Source: CAD feature listing. Evaluate the final solid. Frame: model axes, mm. A direction names the side the tool comes from. Give positions to 0.01 mm unless a question says otherwise; leave off trailing zeros. Order: outer loops, then holes, each group sorted by start corner. A loop starts at its lowest first (then second) coordinate and runs counter-clockwise, first axis right, second up. Notation, with made-up numbers: (87.5, 27) - (121.5, 27) arc R29 cw to (121.5, 63) - close; hole circle Ø4 at (76.5, 73). An arc over 180 degrees is marked (long way). Answer as CSV lines item,"result".
```python
from build123d import *

# Parameters (mm, degrees)
SCHIZZO2_R                    = 10.5
ESTRUSIONE_ESTRUSIONE1_DEPTH  = 22
TAGLIO_ESTRUSIONE1_DEPTH      = 17
SMUSSO1_SIZE                  = 2
TAGLIO_ESTRUSIONE2_DEPTH      = 27.54241888
TAGLIO_ESTRUSIONE2_DEPTH_BACK = 27.54241888
SCHIZZO4_R                    = 2
TAGLIO_ESTRUSIONE3_DEPTH      = 27.542418959
TAGLIO_ESTRUSIONE3_DEPTH_BACK = 19
SCHIZZO5_R                    = 0.9


with BuildPart() as part:
    # Schizzo2 → Estrusione-Estrusione1 (new body)
    with BuildSketch(Plane(origin=(0, 0, 0), x_dir=(1, 0, 0), z_dir=(0, 1, 0))):
        with Locations(Location((0, 0, 0), (0, 0, 270))):
            Circle(SCHIZZO2_R)
    extrude(amount=ESTRUSIONE_ESTRUSIONE1_DEPTH)

    # Schizzo3 → Taglio-Estrusione1 (cut)
    with BuildSketch(Plane.XZ):
        with BuildLine():
            Line((-2.860934268, 7.5), (2.860934268, 7.5))
            ThreePointArc((2.860934268, 7.5), (4.373482153, 6.873482153), (5, 5.360934268))
            Line((5, 5.360934268), (5, -5.360934268))
            ThreePointArc((5, -5.360934268), (4.373482153, -6.873482153), (2.860934268, -7.5))
            Line((2.860934268, -7.5), (-2.860934268, -7.5))
            ThreePointArc((-2.860934268, -7.5), (-4.373482153, -6.873482153), (-5, -5.360934268))
            Line((-5, -5.360934268), (-5, 5.360934268))
            ThreePointArc((-5, 5.360934268), (-4.373482153, 6.873482153), (-2.860934268, 7.5))
        make_face()
    extrude(amount=-TAGLIO_ESTRUSIONE1_DEPTH, mode=Mode.SUBTRACT)

    # Smusso1
    smusso1_edges = [part.edges().sort_by_distance(p)[0] for p in [
        (0, 22, -10.5),
    ]]
    chamfer(smusso1_edges, length=SMUSSO1_SIZE)

    # Schizzo4 → Taglio-Estrusione2 (cut, two sides: drawn at the far end of the back side and taken through both)
    with BuildSketch(Plane(origin=(0, 0, 0), x_dir=(0, 0, -1), z_dir=(1, 0, 0)).offset(-TAGLIO_ESTRUSIONE2_DEPTH_BACK)):
        with Locations(Location((0, 10, 0), (0, 0, 270))):
            Circle(SCHIZZO4_R)
    extrude(amount=TAGLIO_ESTRUSIONE2_DEPTH + TAGLIO_ESTRUSIONE2_DEPTH_BACK, mode=Mode.SUBTRACT)

    # Schizzo5 → Taglio-Estrusione3 (cut, two sides: drawn at the far end of the back side and taken through both)
    with BuildSketch(Plane.XZ.offset(-TAGLIO_ESTRUSIONE3_DEPTH_BACK)):
        with Locations(Location((7, 0, 0), (0, 0, 90))):
            Circle(SCHIZZO5_R)
    extrude(amount=TAGLIO_ESTRUSIONE3_DEPTH + TAGLIO_ESTRUSIONE3_DEPTH_BACK, mode=Mode.SUBTRACT)


solid = part.part
```
(1) Cut plane C-C (x = 0). Return loops of the section in (y, z).
Completed:
outline,"(0, -10.5) - (20, -10.5) - (22, -8.5) - (22, 8.5) - (20, 10.5) - (0, 10.5) - (0, 7.5) - (17, 7.5) - (17, -7.5) - (0, -7.5) - close"
(2) Cut plane D-D (y = 10). Return loops of the section in (x, z).
Completed:
outline,"(-10.31, -2) arc R10.5 ccw to (10.31, -2) - (5, -2) - (5, -5.36) arc R2.14 cw to (2.86, -7.5) - (-2.86, -7.5) arc R2.14 cw to (-5, -5.36) - (-5, -2) - close; (-10.31, 2) - (-5, 2) - (-5, 5.36) arc R2.14 cw to (-2.86, 7.5) - (2.86, 7.5) arc R2.14 cw to (5, 5.36) - (5, 2) - (10.31, 2) arc R10.5 ccw to start"
(3) Mould query, pull axis Z, two halves, no side actions, for faces 3 (the flat face through (0, 17, 0)), 4 (the cylindrical face through (-7.8, 11.6, 1.2)), 5 (the cylindrical face through (-10.25, 9.86, -2.28)), 6 (the flat face through (0, 22, 0)). Classes: released by +Z, released by -Z, zero draft, split by the parting line, or undercut.
Completed:
face 3,"undercut"
face 4,"undercut"
face 5,"split by the parting line"
face 6,"zero draft"
(4) Cut plane B-B (y = 4.75). Return loops of the section in (x, z).
Completed:
outline,"circle Ø21 at (0, 0); hole (-5, -5.36) arc R2.14 ccw to (-2.86, -7.5) - (2.86, -7.5) arc R2.14 ccw to (5, -5.36) - (5, 5.36) arc R2.14 ccw to (2.86, 7.5) - (-2.86, 7.5) arc R2.14 ccw to (-5, 5.36) - close; hole circle Ø1.8 at (7, 0)"
(5) Access query for faces 1 (the cylindrical face through (4.357, 8.381, 6.89)), 2 (the cylindrical face through (7.714, 9.077, 1.774)). Directions: +Z, -Z, +X, -X, +Y, -Y. A direction counts if a zero-diameter tool reaches every point of the face in a straight line with its end or side. Return the directions, or none.
Completed:
face 1,"-Y"
face 2,"+X, -X"
(6) Ray query, line 1 (X direction, y = 4.5, z = 0); line 2 (Y direction, x = 1.75, z = 0.5); line 3 (Z direction, x = 2, y = 10). Return the intervals inside material, ascending. Write a range as from..to.
Completed:
line 1,"-10.5..-5, 5..6.1, 7.9..10.5"
line 2,"17..22"
line 3,"-10.31..-7.5, 7.5..10.31"
(7) Contact query for flat-ended pins moving along their axis: pin 1 (12 mm diameter, centred on y = 10.5, z = 4, fed in from -X); pin 2 (10 mm diameter, centred on y = 13.5, z = -8, fed in from +X); pin 3 (4 mm diameter, centred on x = 6.5, y = 15, fed in from +Z); pin 4 (5 mm diameter, centred on x = -1, z = 0.5, fed in from -Y). Output: stop coordinate, or through.
Completed:
pin 1,"x = -10.5"
pin 2,"x = 10.06"
pin 3,"z = 9.49"
pin 4,"y = 17"
(8) Cut plane A-A (z = 0). Return loops of the section in (x, y), then the cut area to 3 significant figures.
Completed:
outline,"(-10.5, 0) - (-5, 0) - (-5, 8) - (-10.5, 8) - close; (-10.5, 12) - (-5, 12) - (-5, 17) - (5, 17) - (5, 12) - (6.1, 12) - (6.1, 19) - (7.9, 19) - (7.9, 12) - (10.5, 12) - (10.5, 20) - (8.5, 22) - (-8.5, 22) - (-10.5, 20) - close; (5, 0) - (6.1, 0) - (6.1, 8) - (5, 8) - close; (7.9, 0) - (10.5, 0) - (10.5, 8) - (7.9, 8) - close"
area,"217 mm²"
